from build123d import *

# Parameters (mm, degrees)
CROQUIS1_R               = 14.5
MOTOR_DEPTH              = 38
CROQUIS2_R               = 5
SALIENTE_POSTERIOR_DEPTH = 3
BORNES_DEPTH             = 6
CROQUIS4_R               = 0.75
AGUJERO_BORNES_DEPTH     = 25
CROQUIS5_R               = 15
CAJA_REDUCTORA_DEPTH     = 25
CROQUIS6_R               = 2
BRIDA_DEPTH              = 2.5
CROQUIS7_R               = 6.5
SALIENTE_EJE_DEPTH       = 3
CROQUIS8_R               = 3
EJE_DEPTH                = 17
CORTE_PLANO_EJE_DEPTH    = 10
CROQUIS10_R              = 2
CORTE_BRIDA_DEPTH        = 10


with BuildPart() as part:
    # Croquis1 → Motor (new body)
    with BuildSketch(Plane(origin=(0, 0, 0), x_dir=(1, 0, 0), z_dir=(0, 1, 0))):
        Circle(CROQUIS1_R)
    extrude(amount=MOTOR_DEPTH)

    # Croquis2 → Saliente posterior (add)
    with BuildSketch(Plane(origin=(0, 38, 0), x_dir=(1, 0, 0), z_dir=(0, 1, 0))):
        Circle(CROQUIS2_R)
    extrude(amount=SALIENTE_POSTERIOR_DEPTH)

    # Croquis3 → Bornes (add)
    with BuildSketch(Plane(origin=(0, 38, 0), x_dir=(1, 0, 0), z_dir=(0, 1, 0))):
        with BuildLine():
            Line((-2, 9.5), (2, 9.5))
            ThreePointArc((2, 9.5), (2.5, 9), (2, 8.5))
            Line((2, 8.5), (-2, 8.5))
            ThreePointArc((-2, 8.5), (-2.5, 9), (-2, 9.5))
        make_face()
        with BuildLine():
            Line((-2, -9.5), (2, -9.5))
            ThreePointArc((2, -9.5), (2.5, -9), (2, -8.5))
            Line((2, -8.5), (-2, -8.5))
            ThreePointArc((-2, -8.5), (-2.5, -9), (-2, -9.5))
        make_face()
    extrude(amount=BORNES_DEPTH)

    # Croquis4 → Agujero Bornes (cut, through all)
    with BuildSketch(Plane.XY.offset(9.5)):
        with Locations((0, 42)):
            Circle(CROQUIS4_R)
        with BuildLine():
            ThreePointArc((2, 43.866025404), (2.366025404, 43.5), (2.5, 43))
            Line((2.5, 43), (2.5, 44))
            Line((2.5, 44), (2, 44))
            Line((2, 44), (2, 43.866025404))
        make_face()
        with BuildLine():
            ThreePointArc((1.5, 44), (1.758819045, 43.965925826), (2, 43.866025404))
            Line((2, 43.866025404), (2, 44))
            Line((2, 44), (1.5, 44))
        make_face()
        with BuildLine():
            Line((-2, 43.866025404), (-2, 44))
            Line((-2, 44), (-2.5, 44))
            Line((-2.5, 44), (-2.5, 43))
            ThreePointArc((-2.5, 43), (-2.366025404, 43.5), (-2, 43.866025404))
        make_face()
        with BuildLine():
            ThreePointArc((-2, 43.866025404), (-1.758819045, 43.965925826), (-1.5, 44))
            Line((-1.5, 44), (-2, 44))
            Line((-2, 44), (-2, 43.866025404))
        make_face()
    extrude(amount=-AGUJERO_BORNES_DEPTH, mode=Mode.SUBTRACT)

    # Croquis5 → Caja reductora (add)
    with BuildSketch(Plane.XZ):
        Circle(CROQUIS5_R)
    extrude(amount=CAJA_REDUCTORA_DEPTH)

    # Croquis6 → Brida (add)
    with BuildSketch(Plane.XZ.offset(25)):
        with BuildLine():
            Line((-15, 20), (15, 20))
            ThreePointArc((15, 20), (18.535533906, 18.535533906), (20, 15))
            Line((20, 15), (20, -15))
            ThreePointArc((20, -15), (18.535533906, -18.535533906), (15, -20))
            Line((15, -20), (-15, -20))
            ThreePointArc((-15, -20), (-18.535533906, -18.535533906), (-20, -15))
            Line((-20, -15), (-20, 15))
            ThreePointArc((-20, 15), (-18.535533906, 18.535533906), (-15, 20))
        make_face()
        with Locations((-15, 15)):
            Circle(CROQUIS6_R, mode=Mode.SUBTRACT)
        with Locations((15, 15)):
            Circle(CROQUIS6_R, mode=Mode.SUBTRACT)
        with Locations((15, -15)):
            Circle(CROQUIS6_R, mode=Mode.SUBTRACT)
        with Locations((-15, -15)):
            Circle(CROQUIS6_R, mode=Mode.SUBTRACT)
    extrude(amount=BRIDA_DEPTH)

    # Croquis7 → Saliente eje (add)
    with BuildSketch(Plane.XZ.offset(27.5)):
        Circle(CROQUIS7_R)
    extrude(amount=SALIENTE_EJE_DEPTH)

    # Croquis8 → Eje (add)
    with BuildSketch(Plane.XZ.offset(30.5)):
        Circle(CROQUIS8_R)
    extrude(amount=EJE_DEPTH)

    # Croquis9 → Corte Plano eje (cut)
    with BuildSketch(Plane.XZ.offset(47.5)):
        Polygon((-74.796206056, 2), (-2.236067977, 2), (2.236067977, 2), (74.796206056, 2), (74.796206056, 147.120276157), (-74.796206056, 147.120276157), align=None)
    extrude(amount=-CORTE_PLANO_EJE_DEPTH, mode=Mode.SUBTRACT)

    # Croquis10 → Corte Brida (cut)
    with BuildSketch(Plane(origin=(0, -25, 0), x_dir=(1, 0, 0), z_dir=(0, 1, 0))):
        with BuildLine():
            Line((0, 15), (0, 20))
            Line((0, 20), (-15, 20))
            ThreePointArc((-15, 20), (-18.535533906, 18.535533906), (-20, 15))
            Line((-20, 15), (-20, -15))
            ThreePointArc((-20, -15), (-18.535533906, -18.535533906), (-15, -20))
            Line((-15, -20), (0, -20))
            Line((0, -20), (0, -15))
            ThreePointArc((0, -15), (-15, 0), (0, 15))
        make_face()
        with Locations((-15, -15)):
            Circle(CROQUIS10_R, mode=Mode.SUBTRACT)
        with Locations((-15, 15)):
            Circle(CROQUIS10_R, mode=Mode.SUBTRACT)
    extrude(amount=-CORTE_BRIDA_DEPTH, mode=Mode.SUBTRACT)


solid = part.part
Geometry: final body of the model. Coordinates: model frame, mm. A direction names the side the tool comes from. Coordinates: 2 decimals unless noted, no trailing zeros. Order: outer loops, then holes, each group sorted by start corner. A loop starts at its lowest first (then second) coordinate and runs counter-clockwise, first axis right, second up.
(1) Section query B-B (y = 20). Return the cut outline in (x, z).
(2) Section query C-C (y = -19). Return the cut outline in (x, z).
(3) Material intervals for probe 1 along Z at (x, y) = (15, -26.2); probe 2 along X at (y, z) = (42, -9.05); probe 3 along Y at (x, z) = (0, 9.2), sorted ascending.
(4) Draft query along Z for faces 1 (the face through (15, -26, -13)), 2 (the face through (0, 41, 9.5)), 3 (the face through (0, -26, 18)). Return one class per face: pulls with the +Z half, pulls with the -Z half, needs draft (parallel to the pull), parting line crosses it, or undercut.
(5) First-contact query: pin 1 (4.5 mm diameter, centred on x = 0.5, y = 41, fed in from -Z); pin 2 (1.5 mm diameter, centred on x = -2, z = 12, fed in from -Y); pin 3 (3 mm diameter, centred on x = -0.5, y = 42, fed in from +Z). Flat tips, straight axial feed; report the tip coordinate or a pass-through.
(6) Section query A-A (x = -7.5). Return the cut outline in (y, z).
(7) Access query for faces 4 (the face through (0, -43, 2)), 5 (the face through (-0.65, -38.88, -2.93)), 6 (the face through (-14.985, -13.558, 0.66)), 7 (the face through (0, 41, 0)), 8 (the face through (0, -26, -17)). Directions: +Z, -Z, +X, -X, +Y, -Y. A direction counts if a zero-diameter tool reaches every point of the face in a straight line with its end or side. Return the directions, or none.
Solution:
1. outline: circle Ø29 at (0, 0)
2. outline: circle Ø30 at (0, 0)
3. probe 1: z = -20 to -17, -13 to 13, 17 to 20
3. probe 2: x = -2.5 to -0.75, 0.75 to 2.5
3. probe 3: y = -27.5 to 41.25, 42.75 to 44
4. face 1: undercut
4. face 2: pulls with the +Z half
4. face 3: needs draft
5. pin 1: stops at z = -9.5
5. pin 2: stops at y = -27.5
5. pin 3: stops at z = 9.5
6. outline: (-27.5, -12.99) - (0, -12.99) - (0, -12.41) - (38, -12.41) - (38, 12.41) - (0, 12.41) - (0, 12.99) - (-27.5, 12.99) - close
7. face 4: +Z, +X, -X, -Y
7. face 5: -Y
7. face 6: +Y
7. face 7: +X, -X, +Y
7. face 8: -Z, -X, +Y, -Y
